```python
from build123d import *

# Parameters (mm, degrees)
CHAMFER1_SIZE                   = 0.508
CHAMFER2_SIZE                   = 0.254
FILLET1_R                       = 0.762
F_6_32_TAPPED_HOLE1_D           = 2.7051
F_6_32_TAPPED_HOLE1_DEPTH       = 8.07730597
F_6_32_TAPPED_HOLE1_CSINK_D     = 3.81
F_6_32_TAPPED_HOLE1_CSINK_ANGLE = 90
F_6_32_TAPPED_HOLE1_TIP         = 0.81269403
CUT_EXTRUDE1_REACH              = 122.968
SKETCH4_R                       = 4.7625
CHAMFER3_SIZE                   = 0.254
SKETCH5_R                       = 7.9375
CUT_EXTRUDE2_DEPTH              = 9.78408
SKETCH6_R                       = 11.1125
CUT_EXTRUDE3_DEPTH              = 1.5875
CHAMFER4_SIZE                   = 0.508
CUT_EXTRUDE4_DEPTH              = 121.967997999
CUT_EXTRUDE4_DEPTH_BACK         = 121.967997999
SKETCH7_R                       = 2.38125
CUT_EXTRUDE5_DEPTH              = 92.440945536
CUT_EXTRUDE5_DEPTH_BACK         = 1.524
SKETCH8_R                       = 11.1125
SKETCH8_R_2                     = 9.4361
CHAMFER5_SIZE                   = 0.254
SKETCH9_R                       = 7.14375
CUT_EXTRUDE6_DEPTH              = 12.7
CUT_EXTRUDE7_START              = -12.7
SKETCH10_R                      = 7.14375
CUT_EXTRUDE7_DEPTH              = 12.7


with BuildPart() as part:
    # Sketch1 → Revolve1 (revolve)
    with BuildSketch(Plane(origin=(0, 0, 0), x_dir=(1, 0, 0), z_dir=(0, 1, 0)), mode=Mode.PRIVATE) as revolve1_sk:
        Polygon((0, 6.35), (118.491, 6.35), (118.491, 9.3345), (84.328, 9.3345), (84.328, 9.4361), (30.353, 9.4361), (30.353, 15.875), (26.289, 15.875), (26.289, 9.921875), (17.018, 9.921875), (17.018, 12.954), (10.668, 12.954), (10.668, 17.2212), (0, 17.2212), align=None)
    revolve(revolve1_sk.sketch.rotate(Axis((0, 0, 0), (1, 0, 0)), 180), axis=Axis((0, 0, 0), (1, 0, 0)))

    # Chamfer1
    chamfer1_edges = [part.edges().sort_by_distance(p)[0] for p in [
        (118.491, 0, -9.3345),
    ]]
    chamfer(chamfer1_edges, length=CHAMFER1_SIZE)

    # Chamfer2
    chamfer2_edges = [part.edges().sort_by_distance(p)[0] for p in [
        (0, 0, -17.2212),
        (10.668, 0, -17.2212),
        (26.289, 0, -15.875),
        (30.353, 0, -15.875),
    ]]
    chamfer(chamfer2_edges, length=CHAMFER2_SIZE)

    # Fillet1
    fillet1_edges = [part.edges().sort_by_distance(p)[0] for p in [
        (17.018, 0, -12.954),
    ]]
    fillet(fillet1_edges, radius=FILLET1_R)

    # #6-32 Tapped Hole1
    with Locations(Plane.ZY):
        with Locations((0, 15.08125), (15.08125, 0), (0, -15.08125), (-15.08125, 0)):
            CounterSinkHole(F_6_32_TAPPED_HOLE1_D / 2, F_6_32_TAPPED_HOLE1_CSINK_D / 2, depth=F_6_32_TAPPED_HOLE1_DEPTH, counter_sink_angle=F_6_32_TAPPED_HOLE1_CSINK_ANGLE)
            with Locations((0, 0, -(F_6_32_TAPPED_HOLE1_DEPTH + F_6_32_TAPPED_HOLE1_TIP / 2))):  # 118° drill point
                Cone(0, F_6_32_TAPPED_HOLE1_D / 2, F_6_32_TAPPED_HOLE1_TIP, mode=Mode.SUBTRACT)

    # Sketch4 → Cut-Extrude1 (cut, up to next)
    with BuildSketch(Plane.ZY, mode=Mode.PRIVATE) as cut_extrude1_sk1:
        with Locations((-13.470384182, 13.470384182)):
            Circle(SKETCH4_R)
    cut_extrude1_tool1 = extrude(cut_extrude1_sk1.sketch, amount=-CUT_EXTRUDE1_REACH, mode=Mode.PRIVATE) & part.part
    add(cut_extrude1_tool1.solids().sort_by_distance((0, 13.470384, -13.470384))[0], mode=Mode.SUBTRACT)

    # Chamfer3
    # the kernel refuses this chamfer: 0.363987464, 0.254 mm, written as the material it takes off along each edge
    with BuildSketch(Plane(origin=(10.668, 13.470384182, -13.470384182), x_dir=(0, -0.9379671021668624, -0.34672426400916706), z_dir=(0, 0.34672426400916706, -0.9379671021668624))) as chamfer3_piece_1:
        Polygon((4.7625 + CHAMFER3_SIZE, 0), (4.7625, CHAMFER3_SIZE), (4.7625, 0), align=None)
    revolve(axis=Axis((10.668, 13.470384182, -13.470384182), (-1, 0, 0)), revolution_arc=130.574173679, mode=Mode.SUBTRACT)
    with BuildSketch(Plane(origin=(0, 13.470384182, -13.470384182), x_dir=(0, 0.3467242640091905, 0.9379671021668536), z_dir=(-1.1910571492459259e-15, 0.9379671021668536, -0.3467242640091905))) as chamfer3_piece_2:
        Polygon((4.7625 + CHAMFER3_SIZE, 0), (4.7625, CHAMFER3_SIZE), (4.7625, 0), align=None)
    revolve(axis=Axis((0, 13.470384182, -13.470384182), (1, 0, 0)), revolution_arc=130.574173679, mode=Mode.SUBTRACT)
    with BuildSketch(Plane(origin=(11.428728949, 14.75288233, -8.88381632), x_dir=(0, 0.509579415294029, 0.8604236279348654), z_dir=(-1, 0, 0))) as chamfer3_piece_3:
        with BuildLine():
            Line((0.252160633, 0), (-0.117343909, -0.374955046))
            ThreePointArc((-0.117343909, -0.374955046), (-0.056744739, -0.194875402), (0, 0))
            ThreePointArc((0, 0), (0.131188651, 0.00046078), (0.252160633, 0))
        make_face()
    extrude(amount=12.189457898, mode=Mode.SUBTRACT)
    with BuildSketch(Plane(origin=(11.428728949, 8.88381632, -14.75288233), x_dir=(0, -0.8604236279348554, -0.5095794152940455), z_dir=(-1, 0, 0))) as chamfer3_piece_4:
        with BuildLine():
            Line((0.252160633, 0), (-0.117343909, 0.374955046))
            ThreePointArc((-0.117343909, 0.374955046), (-0.056744739, 0.194875402), (0, 0))
            ThreePointArc((0, 0), (0.131188651, -0.00046078), (0.252160633, 0))
        make_face()
    extrude(amount=12.189457898, mode=Mode.SUBTRACT)

    # Sketch5 → Cut-Extrude2 (cut)
    with BuildSketch(Plane.ZY):
        Circle(SKETCH5_R)
    extrude(amount=-CUT_EXTRUDE2_DEPTH, mode=Mode.SUBTRACT)

    # Sketch6 → Cut-Extrude3 (cut)
    with BuildSketch(Plane.ZY):
        Circle(SKETCH6_R)
    extrude(amount=-CUT_EXTRUDE3_DEPTH, mode=Mode.SUBTRACT)

    # Chamfer4
    chamfer4_edges = [part.edges().sort_by_distance(p)[0] for p in [
        (1.5875, 0, -7.9375),
    ]]
    chamfer(chamfer4_edges, length=CHAMFER4_SIZE)

    # Sketch7 → Cut-Extrude4 (cut, two sides: drawn at the far end of the back side and taken through both)
    with BuildSketch(Plane(origin=(0, 0, 0), x_dir=(1, 0, 0), z_dir=(0, 1, 0)).offset(-CUT_EXTRUDE4_DEPTH_BACK)):
        with Locations(Location((86.868, 0, 0), (0, 0, 270))):
            Circle(SKETCH7_R)
    extrude(amount=CUT_EXTRUDE4_DEPTH + CUT_EXTRUDE4_DEPTH_BACK, mode=Mode.SUBTRACT)

    # Sketch8 → Cut-Extrude5 (cut, two sides: drawn at the far end of the back side and taken through both)
    with BuildSketch(Plane(origin=(30.353, 0, 0), x_dir=(0, 0, -1), z_dir=(1, 0, 0)).offset(-CUT_EXTRUDE5_DEPTH_BACK)):
        with Locations(Location((0, 0, 0), (0, 0, 180))):
            Circle(SKETCH8_R)
        with Locations(Location((0, 0, 0), (0, 0, 180))):
            Circle(SKETCH8_R_2, mode=Mode.SUBTRACT)
    extrude(amount=CUT_EXTRUDE5_DEPTH + CUT_EXTRUDE5_DEPTH_BACK, mode=Mode.SUBTRACT)

    # Chamfer5
    chamfer5_edges = [part.edges().sort_by_distance(p)[0] for p in [
        (30.353, 0, -11.1125),
    ]]
    chamfer(chamfer5_edges, length=CHAMFER5_SIZE)

    # Sketch9 → Cut-Extrude6 (cut)
    with BuildSketch(Plane(origin=(118.491, 0, 0), x_dir=(0, 0, -1), z_dir=(1, 0, 0))):
        Circle(SKETCH9_R)
    extrude(amount=-CUT_EXTRUDE6_DEPTH, mode=Mode.SUBTRACT)

    # Sketch10 → Cut-Extrude7 (cut)
    with BuildSketch(Plane.ZY.offset(-9.78408).offset(CUT_EXTRUDE7_START)):
        with Locations(Location((0, 0, 0), (0, 0, 180))):
            Circle(SKETCH10_R)
    extrude(amount=CUT_EXTRUDE7_DEPTH, mode=Mode.SUBTRACT)


solid = part.part
```
Check sheet for the modelled part. Datum: model origin and axes. Units: mm. A direction names the side the tool comes from. Round coordinates to 2 decimals unless told otherwise and drop trailing zeros. Order: outer loops, then holes, each group sorted by start corner. A loop starts at its lowest first (then second) coordinate and runs counter-clockwise, first axis right, second up. Notation, with made-up numbers: (6, 47.25) -> (61, 47.25) arc R19 ccw to (61, 51.25) -> close; hole circle Ø11 at (-19.75, -31.75). An arc over 180 degrees is marked (long way). Use CSV: the item, a comma, the result in double quotes.
(1) Cross-section at B-B (x = 69). Record the boundary of the cut face in (y, z), and give its area (3 significant figures).
Worked out:
outline,"circle Ø18.87 at (0, 0); hole circle Ø12.7 at (0, 0)"
area,"153 mm²"
(2) Cross-section at A-A (x = 101). Record the boundary of the cut face in (y, z), and give its area (3 significant figures).
Worked out:
outline,"circle Ø18.67 at (0, 0); hole circle Ø12.7 at (0, 0)"
area,"147 mm²"
(3) Depth check by flat-ended pin: pin 1 (5 mm diameter, centred on x = 65.5, z = -9, fed in from +Y); pin 2 (2 mm diameter, centred on y = 0, z = -15.08, fed in from -X); pin 3 (15.5 mm diameter, centred on y = 1.5, z = -1, fed in from -X). Enter the tip coordinate at first touch or a pass-through.
Worked out:
pin 1,"y = 6.84"
pin 2,"x = 8.29"
pin 3,"x = 1.59"
(4) Tool access check on faces 1 (the face through (21.589, -2.98, 9.464)), 2 (the face through (5.89, -7.75, -1.72)), 3 (the face through (105.791, -3, 6)). Record the directions out of +Z, -Z, +X, -X, +Y, -Y that give a thin tool (end or side, any length) a straight path to the whole face; none if there is none.
Worked out:
face 1,"none"
face 2,"-X"
face 3,"+X"
(5) Draft check along X on faces 4 (the face through (4.368, 0.059, 16.432)), 5 (the face through (0.13, -11.59, 12.57)), 6 (the face through (89.23, -7.64, -0.31)). Enter one of: pulls with the +X half, pulls with the -X half, needs draft (parallel to the pull), parting line crosses it, or undercut.
Worked out:
face 4,"needs draft"
face 5,"pulls with the -X half"
face 6,"undercut"
(6) Material ranges on line 1 along Y through (x, z) = (5, 0); line 2 along X through (y, z) = (-7, 7.5); line 3 along X through (y, z) = (7.5, -13.5), recorded low to high. Write a range as from..to.
Worked out:
line 1,"-17.22..-16.43, -13.73..-7.94, 7.94..13.73, 16.43..17.22"
line 2,"1.59..17.02, 26.29..28.83"
line 3,"0..10.67, 26.29..30.35"
